Can you work these out from the drawing? Everything is in mm from the part's minimum corner. Give positions to 0.01 mm unless a question says otherwise; leave off trailing zeros. Loops run counter-clockwise (first coordinate to the right, second up) from the corner with the lowest first, then second, coordinate; pieces in that order, holes last.
Q1. If we section it at D-D (z = 5.75): Please give me the cut outline in (x, y).
Q2. If we section it at A-A (z = 19.75): Please give me the cut outline in (x, y).
Q3. If we section it at C-C (y = 0.25): Give the number of separate pieces and of enclosed holes in the cut face, plus the area to 3 significant figures.
Q4. If we section it at B-B (x = 1.5): Please give me the cut outline in (y, z).
Q5. Will this pin go through, and if not, where does the flat tip stop? P1, Ø3.5, axis at x = 8.5, z = 10.5, coming from the -Y side.
Q6. I need wall thicknesses on line 1 (X direction, y = 0.3, z = 19.25); line 2 (X direction, y = 0.4, z = 4); line 3 (Z direction, x = 3.75, y = 0.1). Which ranges of each line are inside material? Lowest first, please.
Q7. We'd pull the mould along X, two halves only. Please class the marked faces 1 and 2: +X half, -X half, draft (parallel to the pull), parting line (faces both ways), or undercut.
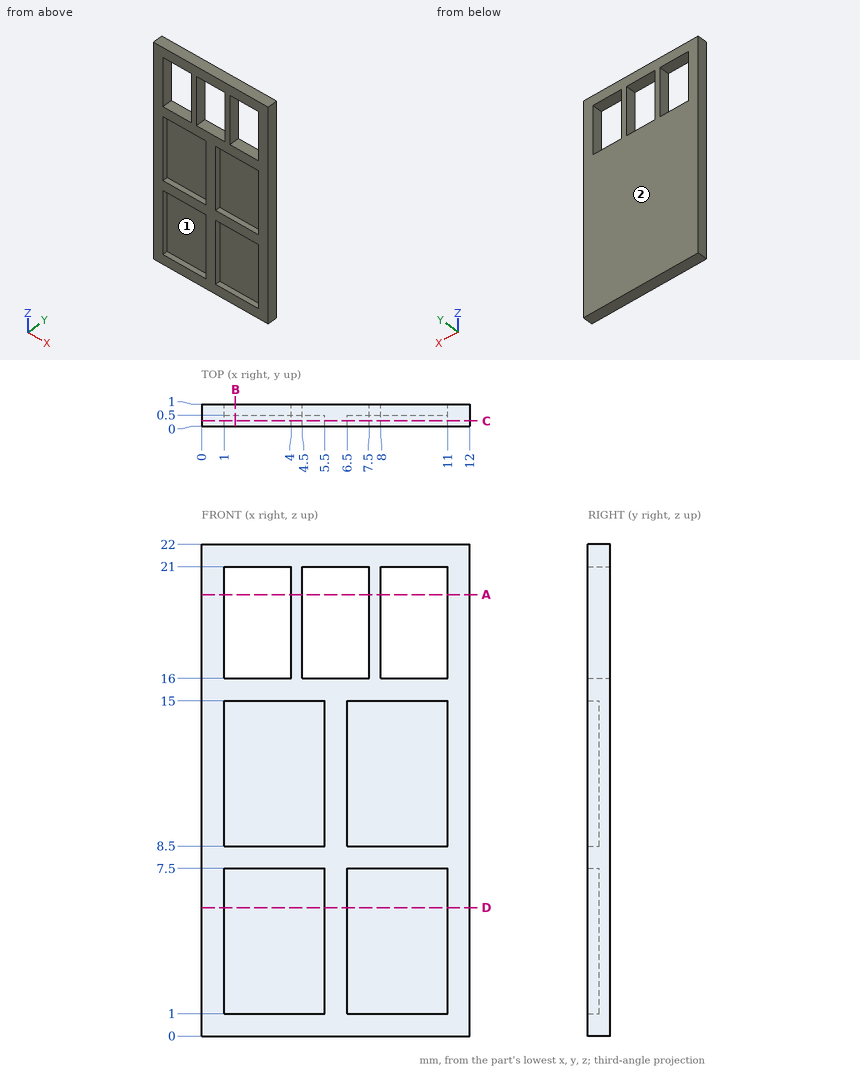
Check sheet entries:
1. outline: (0, 0) - (1, 0) - (1, 0.5) - (5.5, 0.5) - (5.5, 0) - (6.5, 0) - (6.5, 0.5) - (11, 0.5) - (11, 0) - (12, 0) - (12, 1) - (0, 1) - close
2. outline: (0, 0) - (1, 0) - (1, 1) - (0, 1) - close; (4, 0) - (4.5, 0) - (4.5, 1) - (4, 1) - close; (7.5, 0) - (8, 0) - (8, 1) - (7.5, 1) - close; (11, 0) - (12, 0) - (12, 1) - (11, 1) - close
3. separate pieces: 1
3. enclosed holes: 7
3. area: 102 mm2
4. outline: (0, 0) - (1, 0) - (1, 16) - (0, 16) - (0, 15) - (0.5, 15) - (0.5, 8.5) - (0, 8.5) - (0, 7.5) - (0.5, 7.5) - (0.5, 1) - (0, 1) - close; (0, 21) - (1, 21) - (1, 22) - (0, 22) - close
5. P1: stops at y = 0.5
6. line 1: x = 0 to 1, 4 to 4.5, 7.5 to 8, 11 to 12
6. line 2: x = 0 to 1, 5.5 to 6.5, 11 to 12
6. line 3: z = 0 to 1, 7.5 to 8.5, 15 to 16, 21 to 22
7. face 1: undercut
7. face 2: draft
